Design review of the part built by this model. Coordinates are the model's own, in mm. A direction names the side the tool comes from. Coordinates: 2 decimals unless noted, no trailing zeros. Write each loop counter-clockwise with the first axis right and the second up, starting at its lowest first coordinate (ties: lowest second). Pieces come first, ordered by that corner, then holes. Notation, with made-up numbers: M 43,37.25 L 101,37.25 A26 ccw 101,66.25 Z; hole C 63.5,36.5 d9. An arc over 180 degrees is marked long. Write item = value, one per line.
```python
from build123d import *

# Parameters (mm, degrees)
F0_W     = 74.93
F0_H     = 113.284
F1_DEPTH = 7.62
F2_R     = 2.38125
F3_DEPTH = 7.621
F4_R     = 36.322
F5_DEPTH = 36.322


with BuildPart() as f1:
    # F0 (on Front) → F1 (new body)
    with BuildSketch(Plane.XZ):
        Rectangle(F0_W, F0_H)
    extrude(amount=F1_DEPTH)

    # F2 (on face) → F3 (cut, through all)
    with BuildSketch(Plane.XZ.offset(7.62)):
        with Locations((23.876, 41.275)):
            Circle(F2_R)
        with Locations((-23.876, 41.275)):
            Circle(F2_R)
        with Locations((-23.876, -41.275)):
            Circle(F2_R)
        with Locations((23.876, -41.275)):
            Circle(F2_R)
    extrude(amount=-F3_DEPTH, mode=Mode.SUBTRACT)

    # F4 (on face) → F5 (join)
    with BuildSketch(Plane.XZ.offset(7.62)):
        Circle(F4_R)
    extrude(amount=F5_DEPTH)


solid = f1.part
```
Q1. Consider section A-A, the plane z = 0. State the section outline as (x, y) points (3 decimals).
Check result:
outline = M -37.465,-7.62 L -36.322,-7.62 L -36.322,-43.942 L 36.322,-43.942 L 36.322,-7.62 L 37.465,-7.62 L 37.465,0 L -37.465,0 Z
Q2. Machinability: for faces 1 (the cylindrical face through (19.526, -25.527, 30.627)), 2 (the flat face through (-1, 0, 1)), which of the approach directions +Z, -Z, +X, -X, +Y, -Y give a long, thin tool a straight path to every point of the face, cutting with its end or side? Answer none if there is none.
Check result:
face_1 = -Y
face_2 = +Z, -Z, +X, -X, +Y
Q3. The part is to be moulded in two halves that separate along Z. For faces 3 (the cylindrical face through (-21.676, -3.863, -42.187)), 4 (the flat face through (37.465, -4, -1)), 5 (the flat face through (-1, -4, -56.642)), say which applies: +Z half, -Z half, draft (parallel to the pull), parting line (faces both ways), or undercut.
Check result:
face_3 = undercut
face_4 = draft
face_5 = -Z half
Q4. Wall thickness on line 1 (Y direction, x = -20, z = 46); line 2 (X direction, y = -36, z = -31); line 3 (X direction, y = -21, z = 5): over which ranges is each line inside the solid? List them lowest first.
Check result:
line_1 = -7.62 to 0
line_2 = -18.93 to 18.93
line_3 = -35.98 to 35.98
Q5. Consider section B-B, the plane x = 0. State the section outline as (y, z) points.
Check result:
outline = M -43.94,-36.32 L -7.62,-36.32 L -7.62,-56.64 L 0,-56.64 L 0,56.64 L -7.62,56.64 L -7.62,36.32 L -43.94,36.32 Z
Q6. For P1, Ø4, axis at x = 6.5, y = -15.5, coming from the +Z side; P2, Ø2, axis at x = -12.5, z = -12.5, coming from the +Y side; P3, Ø6, axis at x = -21, y = -19.5, coming from the -Z side; P4, Ø1, axis at y = -14, z = -13.5, coming from the -X side, all flat-tipped, find the tip position at first contact; note any pin that passes through.
Check result:
P1 = 36.04
P2 = 0
P3 = -31.55
P4 = -33.92
Q7. Consider section C-C, the plane y = -18.5. State the section outline as (x, z) points, and give its area (3 significant figures).
Check result:
outline = C 0,0 d72.64
area = 4,140 mm²
